from build123d import *

# Parameters (mm, degrees)
CROQUIS1_R              = 100
SALIENTE_EXTRUIR1_DEPTH = 3
CROQUIS3_R              = 110
CORTAR_EXTRUIR1_DEPTH   = 3
REDONDEO1_R             = 10
CROQUIS4_R              = 1.5
CROQUIS4_R_2            = 12.5
CORTAR_EXTRUIR2_DEPTH   = 142.453172607
CROQUIS5_R              = 1.5
CORTAR_EXTRUIR3_DEPTH   = 142.453172607


with BuildPart() as part:
    # Croquis1 → Saliente-Extruir1 (new body)
    with BuildSketch(Plane.XY):
        Circle(CROQUIS1_R)
    extrude(amount=SALIENTE_EXTRUIR1_DEPTH)

    # Croquis3 → Cortar-Extruir1 (cut)
    with BuildSketch(Plane.XY.offset(3)):
        with Locations((190, 0)):
            Circle(CROQUIS3_R)
    extrude(amount=-CORTAR_EXTRUIR1_DEPTH, mode=Mode.SUBTRACT)

    # Redondeo1
    redondeo1_edges = [part.edges().sort_by_distance(p)[0] for p in [
        (89.473684211, -44.659375654, 1.5),
        (89.473684211, 44.659375654, 1.5),
    ]]
    fillet(redondeo1_edges, radius=REDONDEO1_R)

    # Croquis4 → Cortar-Extruir2 (cut, through all)
    with BuildSketch(Plane.XY.offset(3)):
        with Locations((-65.01846853, -38.219121523)):
            Circle(CROQUIS4_R)
        with Locations((-49.462119344, -22.662772337)):
            Circle(CROQUIS4_R)
        with Locations((-22.662772337, -49.462119344)):
            Circle(CROQUIS4_R)
        with Locations((-38.219121523, -65.01846853)):
            Circle(CROQUIS4_R)
        with Locations((-22.662772337, 49.462119344)):
            Circle(CROQUIS4_R)
        with Locations((-38.219121523, 65.01846853)):
            Circle(CROQUIS4_R)
        with Locations((-49.462119344, 22.662772337)):
            Circle(CROQUIS4_R)
        with Locations((-65.01846853, 38.219121523)):
            Circle(CROQUIS4_R)
        with Locations((49.462119344, 22.662772337)):
            Circle(CROQUIS4_R)
        with Locations((65.01846853, 38.219121523)):
            Circle(CROQUIS4_R)
        with Locations((22.662772337, 49.462119344)):
            Circle(CROQUIS4_R)
        with Locations((38.219121523, 65.01846853)):
            Circle(CROQUIS4_R)
        with Locations((22.662772337, -49.462119344)):
            Circle(CROQUIS4_R)
        with Locations((38.219121523, -65.01846853)):
            Circle(CROQUIS4_R)
        with Locations((49.462119344, -22.662772337)):
            Circle(CROQUIS4_R)
        with Locations((65.01846853, -38.219121523)):
            Circle(CROQUIS4_R)
        Circle(CROQUIS4_R_2)
        Polygon((-58.336309448, -83.085046789), (-83.085046789, -58.336309448), (-66.821590822, -42.072853481), (-42.072853481, -66.821590822), align=None)
        Polygon((-66.821590822, 42.072853481), (-42.072853481, 66.821590822), (-58.336309448, 83.085046789), (-83.085046789, 58.336309448), align=None)
        Polygon((42.072853481, 66.821590822), (66.821590822, 42.072853481), (83.085046789, 58.336309448), (58.336309448, 83.085046789), align=None)
        Polygon((66.821590822, -42.072853481), (42.072853481, -66.821590822), (58.336309448, -83.085046789), (83.085046789, -58.336309448), align=None)
    extrude(amount=-CORTAR_EXTRUIR2_DEPTH, mode=Mode.SUBTRACT)

    # Croquis5 → Cortar-Extruir3 (cut, through all)
    with BuildSketch(Plane(origin=(0, 0, 0), x_dir=(-1, 0, 0), z_dir=(0, 0, -1))):
        with Locations((11.5, -90)):
            Circle(CROQUIS5_R)
        with Locations((-11.5, -90)):
            Circle(CROQUIS5_R)
        with Locations((-11.5, -50)):
            Circle(CROQUIS5_R)
        with Locations((11.5, -50)):
            Circle(CROQUIS5_R)
        with Locations((-11.5, 90)):
            Circle(CROQUIS5_R)
        with Locations((11.5, 90)):
            Circle(CROQUIS5_R)
        with Locations((11.5, 50)):
            Circle(CROQUIS5_R)
        with Locations((-11.5, 50)):
            Circle(CROQUIS5_R)
    extrude(amount=-CORTAR_EXTRUIR3_DEPTH, mode=Mode.SUBTRACT)


solid = part.part
Geometry: final body of the model. Coordinates: model frame, mm. A direction names the side the tool comes from. Coordinates: 2 decimals unless noted, no trailing zeros. Order: outer loops, then holes, each group sorted by start corner. A loop starts at its lowest first (then second) coordinate and runs counter-clockwise, first axis right, second up.
(1) Section query A-A (x = 0). Return the cut outline in (y, z), plus the area to 3 significant figures.
(2) Section query B-B (y = 0). Return the cut outline in (x, z).
(3) Access query for faces 1 (the face through (49.55, -74.3, 1.52)), 2 (the face through (-49.55, 74.3, 1.52)), 3 (the face through (74.514, -49.765, 1.521)), 4 (the face through (54.62, -54.274, 1.521)), 5 (the face through (74.3, 49.55, 1.52)). Directions: +Z, -Z, +X, -X, +Y, -Y. A direction counts if a zero-diameter tool reaches every point of the face in a straight line with its end or side. Return the directions, or none.
(4) First-contact query: pin 1 (3.5 mm diameter, centred on x = 11.5, y = -50, fed in from +Z); pin 2 (1.8 mm diameter, centred on x = 22.66, y = 49.46, fed in from +Z); pin 3 (1 mm diameter, centred on x = -73, z = 0.5, fed in from -Y); pin 4 (1 mm diameter, centred on x = 20.5, z = 1.5, fed in from -Y). Flat tips, straight axial feed; report the tip coordinate or a pass-through.
(5) Section query C-C (y = -45.5). State how many separate pieces and enclosed holes the cut face has, plus the area to 3 significant figures.
(6) Draft query along Y for faces 6 (the face through (84.7, 53.16, 1.48)), 7 (the face through (-54.62, 54.274, 1.521)), 8 (the face through (14, 1, 0)). Return one class per face: pulls with the +Y half, pulls with the -Y half, needs draft (parallel to the pull), parting line crosses it, or undercut.
(7) Material intervals for probe 1 along X at (y, z) = (-24, 1.05); probe 2 along X at (y, z) = (-39.5, 1.5); probe 3 along Y at (x, z) = (-11.5, 0.65), sorted ascending.
Solution:
1. outline: (-100, 0) - (-12.5, 0) - (-12.5, 3) - (-100, 3) - close; (12.5, 0) - (100, 0) - (100, 3) - (12.5, 3) - close
1. area: 525 mm2
2. outline: (-100, 0) - (-12.5, 0) - (-12.5, 3) - (-100, 3) - close; (12.5, 0) - (80, 0) - (80, 3) - (12.5, 3) - close
3. face 1: +Z, -Z, +X
3. face 2: +Z, -Z, -X
3. face 3: +Z, -Z, -Y
3. face 4: +Z, -Z
3. face 5: +Z, -Z, +Y
4. pin 1: stops at z = 3
4. pin 2: passes through
4. pin 3: stops at y = -48.75
4. pin 4: stops at y = -97.98
5. separate pieces: 3
5. enclosed holes: 0
5. area: 491 mm2
6. face 6: pulls with the +Y half
6. face 7: undercut
6. face 8: needs draft
7. probe 1: x = -97.08 to -50.14, -48.78 to 48.78, 50.14 to 82.65
7. probe 2: x = -91.87 to -65.8, -64.24 to 64.24, 65.8 to 87.34
7. probe 3: y = -99.34 to -91.5, -88.5 to -51.5, -48.5 to -4.9, 4.9 to 48.5, 51.5 to 88.5, 91.5 to 99.34
